Work out the finished part from the listing and answer in its coordinate system (mm). Face numbers are marked on the shaded views. A direction names the side the tool comes from. Round coordinates to 2 decimals unless told otherwise and drop trailing zeros. Write each loop counter-clockwise with the first axis right and the second up, starting at its lowest first coordinate (ties: lowest second). Pieces come first, ordered by that corner, then holes.
from build123d import *

# Parameters (mm, degrees)
SKETCH_W     = 28
SKETCH_H     = 21
PAD_DEPTH    = 3
SKETCH001_W  = 28
SKETCH001_H  = 9
PAD001_DEPTH = 2
SKETCH002_R  = 1.6
POCKET_DEPTH = 3.001
FILLET_R     = 1
FILLET001_R  = 1
FILLET002_R  = 1
FILLET003_R  = 1


with BuildPart() as part:
    # Sketch → Pad (new body)
    with BuildSketch(Plane.XY):
        with Locations((14, 10.5)):
            Rectangle(SKETCH_W, SKETCH_H)
    extrude(amount=PAD_DEPTH)

    # Sketch001 (on Face6 of Pad) → Pad001 (join)
    with BuildSketch(Plane.XY.offset(3)):
        with Locations((14, 10.5)):
            Rectangle(SKETCH001_W, SKETCH001_H)
    extrude(amount=PAD001_DEPTH)

    # Sketch002 (on Face5 of Pad001) → Pocket (cut, through all)
    with BuildSketch(Plane.XY.offset(3)):
        with Locations((3.5, 3)):
            Circle(SKETCH002_R)
        with Locations((24.5, 3)):
            Circle(SKETCH002_R)
        with Locations((3.5, 18)):
            Circle(SKETCH002_R)
        with Locations((24.5, 18)):
            Circle(SKETCH002_R)
    extrude(amount=-POCKET_DEPTH, mode=Mode.SUBTRACT)

    # Fillet
    fillet_edges = [part.edges().sort_by_distance(p)[0] for p in [
        (28, 0, 1.5),
        (28, 21, 1.5),
        (0, 0, 1.5),
        (0, 21, 1.5),
    ]]
    fillet(fillet_edges, radius=FILLET_R)

    # Fillet001
    fillet001_edges = [part.edges().sort_by_distance(p)[0] for p in [
        (0, 6, 4),
    ]]
    fillet(fillet001_edges, radius=FILLET001_R)

    # Fillet002
    fillet002_edges = [part.edges().sort_by_distance(p)[0] for p in [
        (28, 6, 4),
    ]]
    fillet(fillet002_edges, radius=FILLET002_R)

    # Fillet003
    fillet003_edges = [part.edges().sort_by_distance(p)[0] for p in [
        (0, 15, 4),
        (28, 15, 4),
    ]]
    fillet(fillet003_edges, radius=FILLET003_R)


solid = part.part
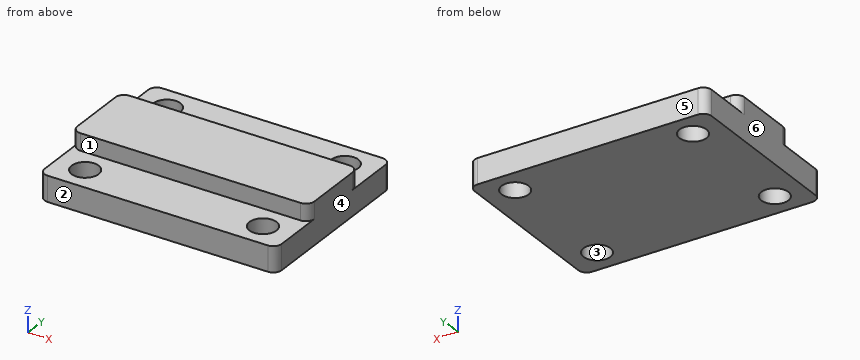
Q1. Find section A-A (x = 24.5). Determine the outline of the cut face in (y, z).
Q2. Find section D-D (x = 9.75). Determine the outline of the cut face in (y, z), plus the area to 3 significant figures.
Q3. Find the intervals of material crossed by L1, parallel to Y at x = 3.5, z = 1.15; L2, parallel to X at y = 19, z = 1.95; L3, parallel to X at y = 4.25, z = 1, in increasing order.
Q4. A tool of negligible diameter and unlimited length cuts with its end or side. For the marked faces 1 and 2, from which of +Z, -Z, +X, -X, +Y, -Y can it reach the whole face along a straight path? Write none if from no direction.
Q5. Find section B-B (y = 18). Determine the outline of the cut face in (x, z), plus the area to 3 significant figures.
Q6. The mould has two halves that part along X. Classify the marked faces 3, 4, 5 and 6: +X half, -X half, draft (parallel to the pull), parting line (faces both ways), or undercut.
Q7. Find section C-C (z = 0.45). Determine the outline of the cut face in (x, y), plus the area to 3 significant figures.
Q8. Given pin 1 (4 mm diameter, centred on x = 8.5, y = 17, fed in from -Z); pin 2 (1 mm diameter, centred on x = 7.5, z = 4, fed in from -Y); pin 3 (3.5 mm diameter, centred on x = 10.5, y = 2.5, fed in from +Z); pin 4 (1.5 mm diameter, centred on y = 6, z = 4.5, fed in from -X), each flat-ended and moving along its own axis, determine where each tip first touches the part or whether it passes through.
Report:
1. outline: (0, 0) - (1.4, 0) - (1.4, 3) - (0, 3) - close; (4.6, 0) - (16.4, 0) - (16.4, 3) - (15, 3) - (15, 5) - (6, 5) - (6, 3) - (4.6, 3) - close; (19.6, 0) - (21, 0) - (21, 3) - (19.6, 3) - close
2. outline: (0, 0) - (21, 0) - (21, 3) - (15, 3) - (15, 5) - (6, 5) - (6, 3) - (0, 3) - close
2. area: 81.0 mm2
3. L1: y = 0 to 1.4, 4.6 to 16.4, 19.6 to 21
3. L2: x = 0 to 2.25, 4.75 to 23.25, 25.75 to 28
3. L3: x = 0 to 2.5, 4.5 to 23.5, 25.5 to 28
4. face 1: +Z, +X, -X, -Y
4. face 2: +Z, -Z, +X, -X, -Y
5. outline: (0, 0) - (1.9, 0) - (1.9, 3) - (0, 3) - close; (5.1, 0) - (22.9, 0) - (22.9, 3) - (5.1, 3) - close; (26.1, 0) - (28, 0) - (28, 3) - (26.1, 3) - close
5. area: 64.8 mm2
6. face 3: undercut
6. face 4: +X half
6. face 5: draft
6. face 6: -X half
7. outline: (0, 1) arc R1 ccw to (1, 0) - (27, 0) arc R1 ccw to (28, 1) - (28, 20) arc R1 ccw to (27, 21) - (1, 21) arc R1 ccw to (0, 20) - close; hole circle Ø3.2 at (3.5, 3); hole circle Ø3.2 at (3.5, 18); hole circle Ø3.2 at (24.5, 3); hole circle Ø3.2 at (24.5, 18)
7. area: 555 mm2
8. pin 1: stops at z = 0
8. pin 2: stops at y = 6
8. pin 3: stops at z = 3
8. pin 4: stops at x = 0.03
